Here's the drawing with two shaded views (mm, measured from the low corner). I have some questions. Coordinates: 2 decimals unless noted, no trailing zeros. Write each loop counter-clockwise with the first axis right and the second up, starting at its lowest first coordinate (ties: lowest second). Pieces come first, ordered by that corner, then holes.
Item 1: I want a section at B-B on y = 7.14. State how many separate pieces and enclosed holes the cut face has, then the cut area to 3 significant figures.
Item 2: If I drill on probe 1 along Y at (x, z) = (4.5, 1.1); probe 2 along X at (y, z) = (6.75, 6.25); probe 3 along Z at (x, y) = (58.5, 5.75), over which ranges is the centre line in solid material (lowest first)?
Item 3: I want a section at A-A on x = 46.1. Please give me the cut outline in (y, z), then the cut area to 3 significant figures.
Item 4: For P1, Ø5, axis at x = 63.5, y = 12, coming from the +Z side; P2, Ø5, axis at x = 25.5, z = 8, coming from the -Y side; P3, Ø1.8, axis at x = 4.5, y = 7.14, coming from the -Z side, each with a flat end and sliding along its axis, tell me the tip position at first contact or that it passes through.
Item 5: I want a section at C-C on z = 9.25. Please give me the cut outline in (x, y), then the cut area to 3 significant figures.
Item 6: I want a section at D-D on z = 2.75. Please give me the cut outline in (x, y), then the cut area to 3 significant figures.
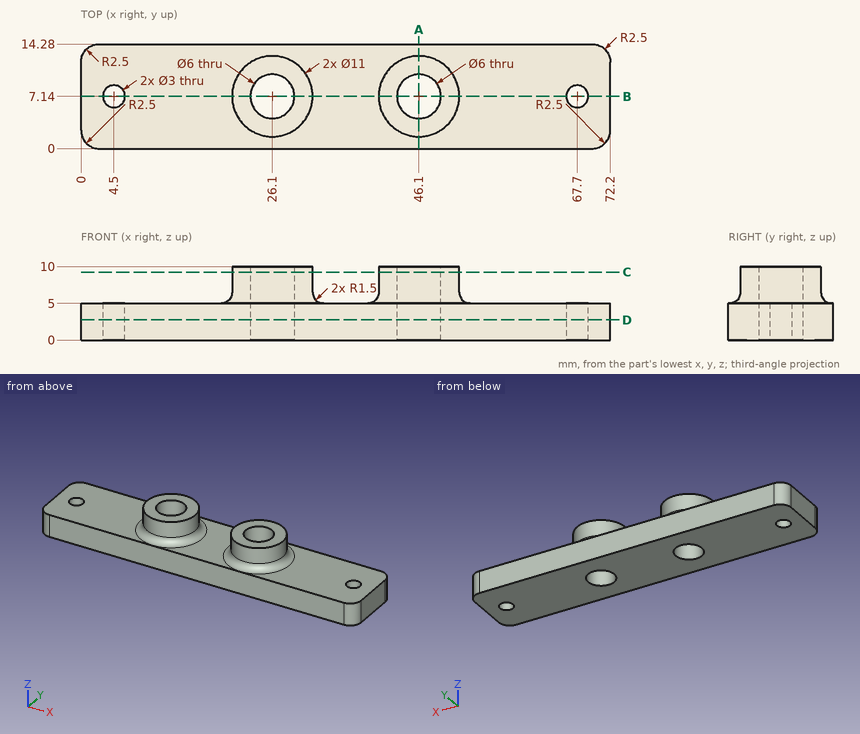
Response values:
1. separate pieces: 5
1. enclosed holes: 0
1. area: 323 mm2
2. probe 1: y = 0 to 5.64, 8.64 to 14.28
2. probe 2: x = 20.59 to 23.13, 29.07 to 31.61, 40.59 to 43.13, 49.07 to 51.61
2. probe 3: z = 0 to 5
3. outline: (0, 0) - (4.14, 0) - (4.14, 10) - (1.64, 10) - (1.64, 6.5) arc R1.5 cw to (0.14, 5) - (0, 5) - close; (10.14, 0) - (14.28, 0) - (14.28, 5) - (14.14, 5) arc R1.5 cw to (12.64, 6.5) - (12.64, 10) - (10.14, 10) - close
3. area: 67.4 mm2
4. P1: stops at z = 5
4. P2: stops at y = 1.28
4. P3: passes through
5. outline: circle Ø11 at (26.1, 7.14); circle Ø11 at (46.1, 7.14); hole circle Ø6 at (26.1, 7.14); hole circle Ø6 at (46.1, 7.14)
5. area: 134 mm2
6. outline: (0, 2.5) arc R2.5 ccw to (2.5, 0) - (69.7, 0) arc R2.5 ccw to (72.2, 2.5) - (72.2, 11.78) arc R2.5 ccw to (69.7, 14.28) - (2.5, 14.28) arc R2.5 ccw to (0, 11.78) - close; hole circle Ø3 at (4.5, 7.14); hole circle Ø6 at (26.1, 7.14); hole circle Ø6 at (46.1, 7.14); hole circle Ø3 at (67.7, 7.14)
6. area: 955 mm2
